Here's the drawing with two shaded views (mm, measured from the low corner). I have some questions. Coordinates: 2 decimals unless noted, no trailing zeros. Write each loop counter-clockwise with the first axis right and the second up, starting at its lowest first coordinate (ties: lowest second). Pieces come first, ordered by that corner, then holes. Notation, with made-up numbers: M 82.25,51 L 103.25,51 A11 cw 103.25,67 Z; hole C -2.5,-29.5 d8. An arc over 180 degrees is marked long. Use one line per item in the form item = value. Start each with the question number.
1. I'm going to push a flat-ended pin straight in: pin 1 Ø0.5 at (x, z) = (59.5, 0.5) entering from -Y. Where does the tip first touch, or does it pass through?
2. I want a section at B-B, the plane y = 2. List the corners of the cut face in (x, z) for me, plus the area to 3 significant figures.
3. I want a section at C-C, the plane x = 12.5. List the corners of the cut face in (y, z) for me.
4. I want a section at A-A, the plane z = 0.5. List the corners of the cut face in (x, y) for me, plus the area to 3 significant figures.
5. Please list where these lines run through material, in increasing order: line 1 along Y through (x, z) = (22.5, 0.9); line 2 along Y through (x, z) = (26, 0.1). Write a range as [from, to].
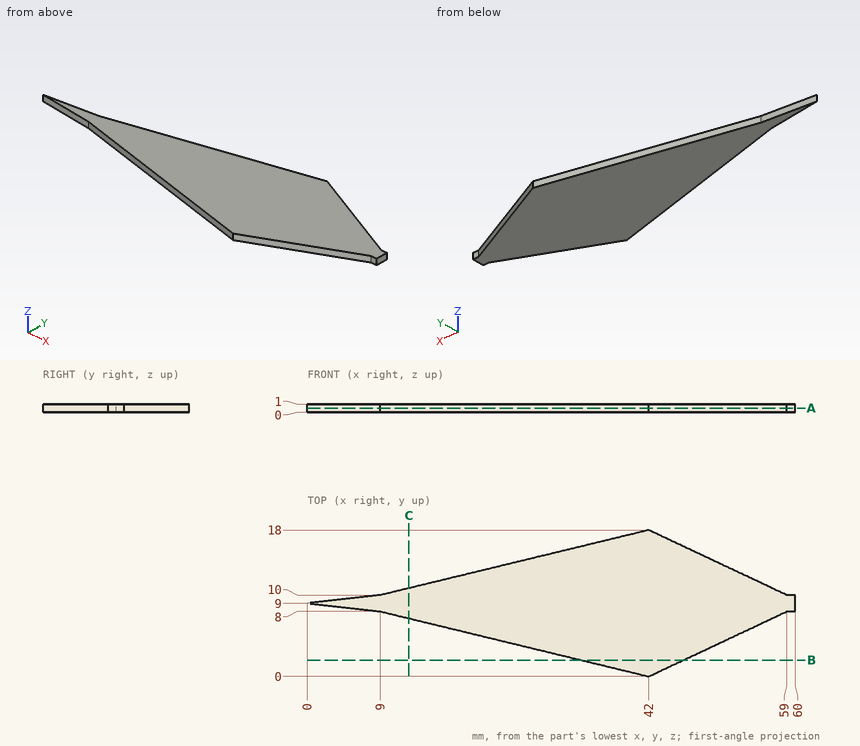
Answer list:
q1.pin_1 = 8
q2.outline = M 33.75,0 L 46.25,0 L 46.25,1 L 33.75,1 Z
q2.area = 12.5 mm²
q3.outline = M 7.15,0 L 10.85,0 L 10.85,1 L 7.15,1 Z
q4.outline = M 0,9 L 9,8 L 42,0 L 59,8 L 60,8 L 60,10 L 59,10 L 42,18 L 9,10 Z
q4.area = 511 mm²
q5.line_1 = [4.73, 13.27]
q5.line_2 = [3.88, 14.12]
